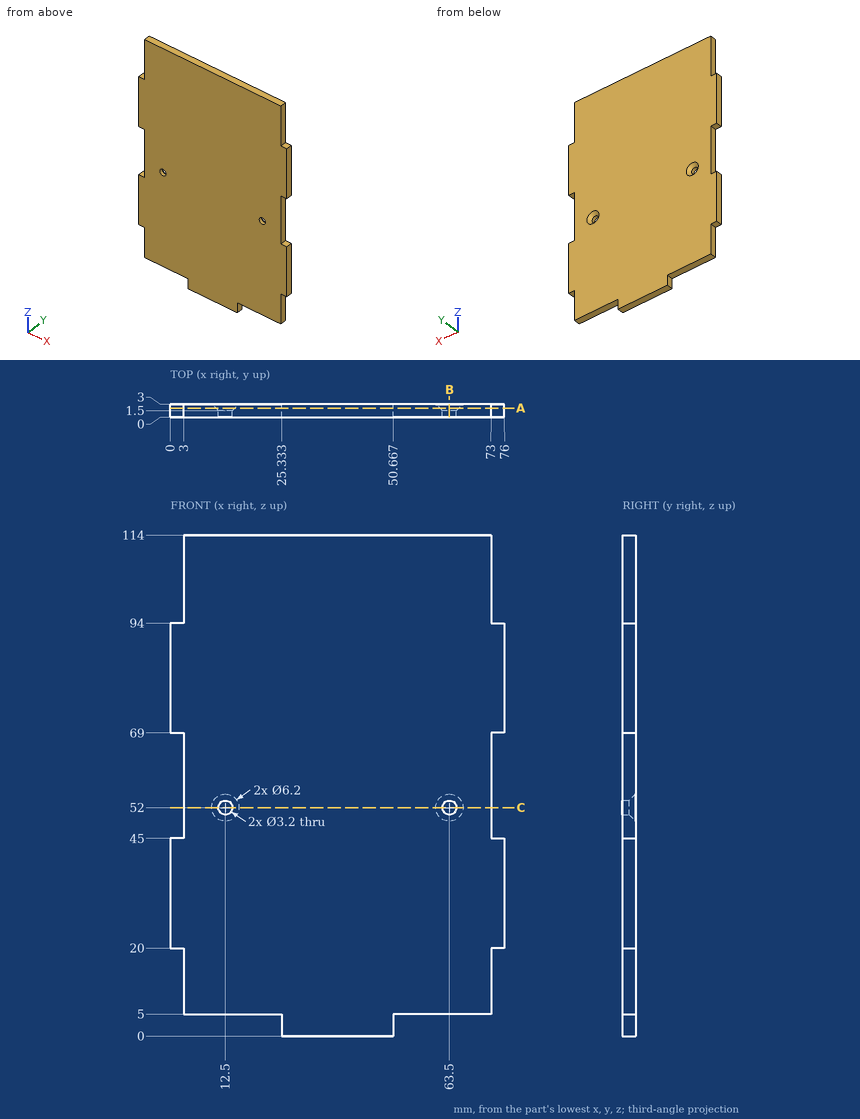
For this review, use the dimensioned drawing (mm, ordinates from the lowest corner) and the shaded views. Coordinates: 2 decimals unless noted, no trailing zeros. Loops run counter-clockwise (first coordinate to the right, second up) from the corner with the lowest first, then second, coordinate; pieces in that order, holes last. Notation, with made-up numbers: (72.25, 54.25) -> (87.25, 54.25) arc R14 ccw to (87.25, 70.25) -> close; hole circle Ø7 at (-22.5, 18). An arc over 180 degrees is marked (long way). Return JSON: item names as keys, results as strings. Group by question number.
(1) Consider section C-C, the plane z = 52. Give the boundary of the cut face in (x, y), plus the area to 3 significant figures.
(2) To check wall thickness, follow L1, parallel to X at y = 0.4, z = 52; L2, parallel to X at y = 0.65, z = 109; L3, parallel to Z at x = 60, y = 1.7. State the ranges of each line that lie inside material, in increasing order.
(3) Consider section A-A, the plane y = 2.05. Give the boundary of the cut face in (x, z), plus the area to 3 significant figures.
(4) Consider section B-B, the plane x = 63.5. Give the boundary of the cut face in (y, z), plus the area to 3 significant figures.
(5) For pin 1 Ø1.5 at (x, y) = (74, 1.5) entering from -Z; pin 2 Ø0.9 at (x, y) = (18, 1) entering from -Z; pin 3 Ø0.9 at (y, z) = (1.5, 101.5) entering from +X, all flat-tipped, find the tip position at first contact; note any pin that passes through.
Results below:
{
 "1": {"outline": "(3, 0) -> (10.9, 0) -> (10.9, 1.5) -> (9.4, 3) -> (3, 3) -> close; (14.1, 0) -> (61.9, 0) -> (61.9, 1.5) -> (60.4, 3) -> (15.6, 3) -> (14.1, 1.5) -> close; (65.1, 0) -> (73, 0) -> (73, 3) -> (66.6, 3) -> (65.1, 1.5) -> close", "area": "186 mm2"},
 "2": {"L1": "x = 3 to 10.9, 14.1 to 61.9, 65.1 to 73", "L2": "x = 3 to 73", "L3": "z = 5 to 114"},
 "3": {"outline": "(0, 20) -> (3, 20) -> (3, 5) -> (25.33, 5) -> (25.33, 0) -> (50.67, 0) -> (50.67, 5) -> (73, 5) -> (73, 20) -> (76, 20) -> (76, 45) -> (73, 45) -> (73, 69) -> (76, 69) -> (76, 94) -> (73, 94) -> (73, 114) -> (3, 114) -> (3, 94) -> (0, 94) -> (0, 69) -> (3, 69) -> (3, 45) -> (0, 45) -> close; hole circle Ø4.3 at (12.5, 52); hole circle Ø4.3 at (63.5, 52)", "area": "8,030 mm2"},
 "4": {"outline": "(0, 5) -> (3, 5) -> (3, 48.9) -> (1.5, 50.4) -> (0, 50.4) -> close; (0, 53.6) -> (1.5, 53.6) -> (3, 55.1) -> (3, 114) -> (0, 114) -> close", "area": "315 mm2"},
 "5": {"pin 1": "stops at z = 20", "pin 2": "stops at z = 5", "pin 3": "stops at x = 73"}
}
